```python
from build123d import *

# Parameters (mm, degrees)
SKETCH1_W           = 200
SKETCH1_H           = 50
BOSS_EXTRUDE1_DEPTH = 10
SKETCH2_R           = 5
SKETCH2_R_2         = 3
SKETCH2_R_3         = 4.25
CUT_EXTRUDE1_DEPTH  = 104.561575886
SKETCH3_R           = 3.4
CUT_EXTRUDE2_DEPTH  = 104.561575886


with BuildPart() as part:
    # Sketch1 → Boss-Extrude1 (new body)
    with BuildSketch(Plane.XY):
        Rectangle(SKETCH1_W, SKETCH1_H)
    extrude(amount=BOSS_EXTRUDE1_DEPTH)

    # Sketch2 → Cut-Extrude1 (cut, through all)
    with BuildSketch(Plane.XY.offset(10)):
        with Locations((90, 10)):
            Circle(SKETCH2_R)
        with Locations((2.5, 10)):
            Circle(SKETCH2_R_2)
        with Locations((-37.5, 17)):
            Circle(SKETCH2_R_2)
        with Locations((-37.5, 3)):
            Circle(SKETCH2_R_3)
    extrude(amount=-CUT_EXTRUDE1_DEPTH, mode=Mode.SUBTRACT)

    # Sketch3 → Cut-Extrude2 (cut, through all)
    with BuildSketch(Plane.XY.offset(10)):
        with Locations((-89.5, -15)):
            Circle(SKETCH3_R)
        with Locations((70, -15)):
            Circle(SKETCH3_R)
        with Locations((85, -15)):
            Circle(SKETCH3_R)
    extrude(amount=-CUT_EXTRUDE2_DEPTH, mode=Mode.SUBTRACT)


solid = part.part
```
Geometry: final body of the model. Coordinates: model frame, mm. Round coordinates to 2 decimals unless told otherwise and drop trailing zeros. Order: outer loops, then holes, each group sorted by start corner. A loop starts at its lowest first (then second) coordinate and runs counter-clockwise, first axis right, second up. Notation, with made-up numbers: (-20.5, -2.75) - (17.5, -2.75) arc R21 cw to (17.5, 2.25) - close; hole circle Ø4 at (5.25, 47.5). An arc over 180 degrees is marked (long way). Write item = value, one per line. Start each with the question number.
Q1. Cut plane D-D on x = -89.5. Return the cut outline in (y, z), and give its area (3 significant figures).
Q2. Pull-direction query (Y, two-part tool) for faces 1 (the flat face through (-1, 25, 5)), 2 (the flat face through (100, 0, 5)), 3 (the cylindrical face through (-41.746, 3.187, 5.07)); classes: +Y half, -Y half, draft (parallel to the pull), parting line (faces both ways), or undercut.
Q3. Cut plane B-B on y = 17. Return the cut outline in (x, z), and give its area (3 significant figures).
Q4. Pin query (flat end, axial travel): pin 1 (10 mm diameter, centred on x = -37.5, y = 3, fed in from +Z); pin 2 (5.5 mm diameter, centred on x = -37.5, y = 17, fed in from -Z). Return the tip coordinate at first contact, or that it passes through.
Q5. Cut plane C-C on x = -37.5. Return the cut outline in (y, z).
Q6. Cut plane A-A on z = 6.25. Return the cut outline in (x, y), and give its area (3 significant figures).
Q7. Ray query, line 1 (Y direction, x = -37.5, z = 3.25); line 2 (Y direction, x = 90, z = 4.75); line 3 (X direction, y = 8, z = 5.5). Return the intervals inside material, ascending. Write a range as from..to.
Outcome:
q1.outline = (-25, 0) - (-18.4, 0) - (-18.4, 10) - (-25, 10) - close; (-11.6, 0) - (25, 0) - (25, 10) - (-11.6, 10) - close
q1.area = 432 mm^2
q2.face_1 = +Y half
q2.face_2 = draft
q2.face_3 = undercut
q3.outline = (-100, 0) - (-40.5, 0) - (-40.5, 10) - (-100, 10) - close; (-34.5, 0) - (100, 0) - (100, 10) - (-34.5, 10) - close
q3.area = 1,940 mm^2
q4.pin_1 = 10
q4.pin_2 = through
q5.outline = (-25, 0) - (-1.25, 0) - (-1.25, 10) - (-25, 10) - close; (7.25, 0) - (14, 0) - (14, 10) - (7.25, 10) - close; (20, 0) - (25, 0) - (25, 10) - (20, 10) - close
q6.outline = (-100, -25) - (100, -25) - (100, 25) - (-100, 25) - close; hole circle Ø6.8 at (-89.5, -15); hole circle Ø8.5 at (-37.5, 3); hole circle Ø6 at (-37.5, 17); hole circle Ø6 at (2.5, 10); hole circle Ø6.8 at (70, -15); hole circle Ø6.8 at (85, -15); hole circle Ø10 at (90, 10)
q6.area = 9,700 mm^2
q7.line_1 = -25..-1.25, 7.25..14, 20..25
q7.line_2 = -25..5, 15..25
q7.line_3 = -100..0.26, 4.74..85.42, 94.58..100
